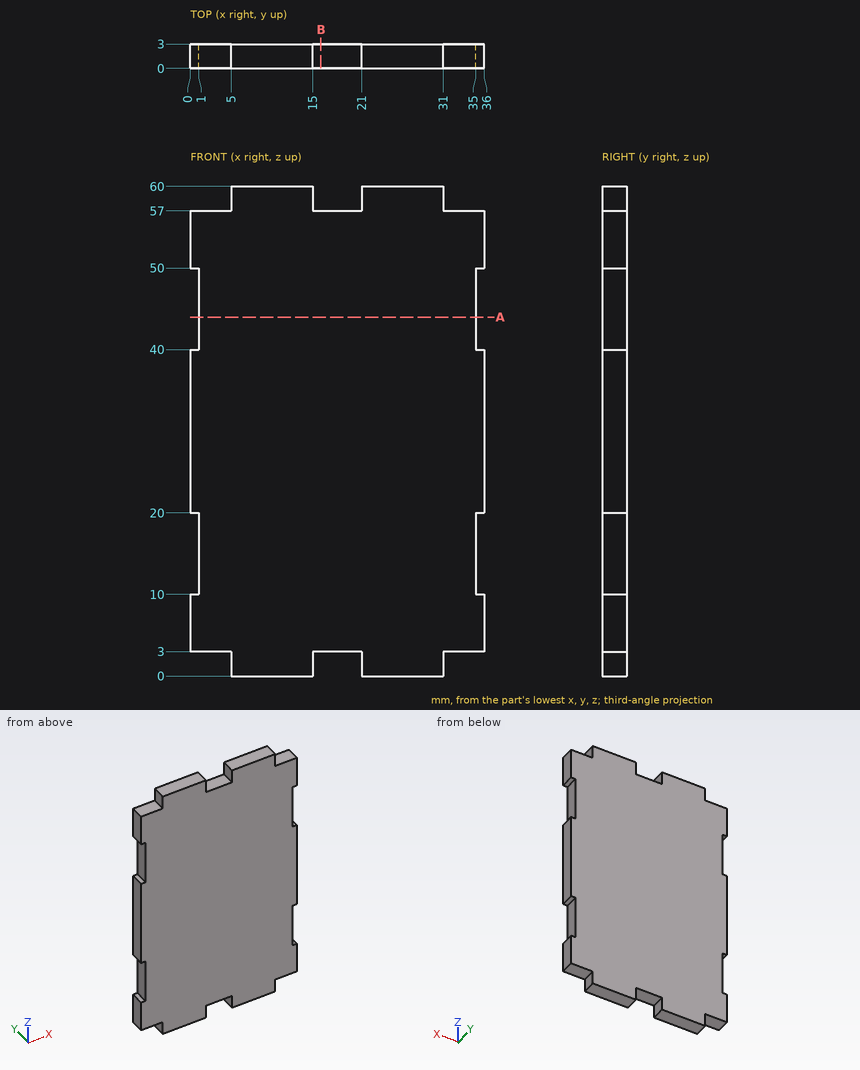
Drawing for the job (mm, zero at the part's lowest x, y, z). Round coordinates to 2 decimals unless told otherwise and drop trailing zeros. Loops run counter-clockwise (first coordinate to the right, second up) from the corner with the lowest first, then second, coordinate; pieces in that order, holes last. Notation, with made-up numbers: (-6, 42.25) -> (12, 42.25) arc R34 ccw to (12, 73.25) -> close; hole circle Ø8 at (51.25, 13). An arc over 180 degrees is marked (long way). Use one line per item in the form item = value. Start each with the question number.
Item 1: Drill centre lines: line 1 along X through (y, z) = (0.8, 41.5); line 2 along Z through (x, y) = (18, 1.7). Where is each one in solid material? Low to high.
Item 2: Band-saw the part on B-B (x = 16). List the corners of the cut face in (y, z), plus the area to 3 significant figures.
Item 3: Band-saw the part on A-A (z = 44). List the corners of the cut face in (x, y).
Item 4: Drop flat-ended pins along their axis: pin 1 Ø0.9 at (y, z) = (2, 44) entering from -X; pin 2 Ø1.5 at (y, z) = (1.5, 1.5) entering from -X; pin 3 Ø0.8 at (x, y) = (35.5, 2) entering from +Z. Give the stop position or say it passes through.
Data:
q1.line_1 = 1 to 35
q1.line_2 = 3 to 57
q2.outline = (0, 3) -> (3, 3) -> (3, 57) -> (0, 57) -> close
q2.area = 162 mm^2
q3.outline = (1, 0) -> (35, 0) -> (35, 3) -> (1, 3) -> close
q4.pin_1 = 1
q4.pin_2 = 5
q4.pin_3 = 57
